from build123d import *

# Parameters (mm, degrees)
BOSS_EXTRUDE2_DEPTH   = 6.35
BOSS_EXTRUDE2_2_DEPTH = 6.35
BOSS_EXTRUDE3_DEPTH   = 12.7
CUT_EXTRUDE2_REACH    = 189.943
SKETCH3_R             = 1.397
CUT_EXTRUDE3_REACH    = 184.986
SKETCH4_R             = 1.35255
SKETCH5_R             = 1.75
CUT_EXTRUDE5_DEPTH    = 24


with BuildPart() as part:
    # Sketch1 → Boss-Extrude2 (new body)
    with BuildSketch(Plane(origin=(0, 0, 0), x_dir=(1, 0, 0), z_dir=(0, 1, 0))):
        Polygon((12.7, 68.58), (40.64, 68.58), (40.64, 78.74), (0, 78.74), (0, 12.7), (12.7, 12.7), align=None)
    extrude(amount=BOSS_EXTRUDE2_DEPTH)



with BuildPart() as body_2:
    # Sketch1 → Boss-Extrude2 2 (new body)
    with BuildSketch(Plane(origin=(0, 0, 0), x_dir=(1, 0, 0), z_dir=(0, 1, 0))):
        Polygon((157.48, 68.58), (157.48, 12.7), (170.18, 12.7), (170.18, 78.74), (129.54, 78.74), (129.54, 68.58), align=None)
    extrude(amount=BOSS_EXTRUDE2_2_DEPTH)


with BuildPart() as part_1:
    add(part.part)

    add(body_2.part)  # Boss-Extrude3 merges body 2
    # Sketch1_3 → Boss-Extrude3 (add)
    with BuildSketch(Plane(origin=(0, 0, 0), x_dir=(1, 0, 0), z_dir=(0, 1, 0))):
        Polygon((157.48, 12.7), (12.7, 12.7), (0, 12.7), (0, 0), (170.18, 0), (170.18, 12.7), align=None)
    extrude(amount=BOSS_EXTRUDE3_DEPTH)

    # Sketch3 → Cut-Extrude2 (cut, up to next)
    with BuildSketch(Plane(origin=(0, 12.7, 0), x_dir=(1, 0, 0), z_dir=(0, 1, 0)), mode=Mode.PRIVATE) as cut_extrude2_sk1:
        with Locations(Location((75.565, 4.7625, 0), (0, 0, 270))):
            Circle(SKETCH3_R)
    cut_extrude2_tool1 = extrude(cut_extrude2_sk1.sketch, amount=-CUT_EXTRUDE2_REACH, mode=Mode.PRIVATE) & part_1.part
    # Sketch3 → Cut-Extrude2 (cut, up to next)
    with BuildSketch(Plane(origin=(0, 12.7, 0), x_dir=(1, 0, 0), z_dir=(0, 1, 0)), mode=Mode.PRIVATE) as cut_extrude2_sk2:
        with Locations(Location((94.615, 7.9375, 0), (0, 0, 270))):
            Circle(SKETCH3_R)
    cut_extrude2_tool2 = extrude(cut_extrude2_sk2.sketch, amount=-CUT_EXTRUDE2_REACH, mode=Mode.PRIVATE) & part_1.part
    add(cut_extrude2_tool1.solids().sort_by_distance((75.565, 12.7, -4.7625))[0], mode=Mode.SUBTRACT)
    add(cut_extrude2_tool2.solids().sort_by_distance((94.615, 12.7, -7.9375))[0], mode=Mode.SUBTRACT)

    # Sketch4 → Cut-Extrude3 (cut, up to next)
    with BuildSketch(Plane(origin=(0, 0, -12.7), x_dir=(-1, 0, 0), z_dir=(0, 0, -1)), mode=Mode.PRIVATE) as cut_extrude3_sk1:
        with Locations((-87.4776, 3.175)):
            Circle(SKETCH4_R)
    cut_extrude3_tool1 = extrude(cut_extrude3_sk1.sketch, amount=-CUT_EXTRUDE3_REACH, mode=Mode.PRIVATE) & part_1.part
    # Sketch4 → Cut-Extrude3 (cut, up to next)
    with BuildSketch(Plane(origin=(0, 0, -12.7), x_dir=(-1, 0, 0), z_dir=(0, 0, -1)), mode=Mode.PRIVATE) as cut_extrude3_sk2:
        with Locations((-79.546452542, 9.525)):
            Circle(SKETCH4_R)
    cut_extrude3_tool2 = extrude(cut_extrude3_sk2.sketch, amount=-CUT_EXTRUDE3_REACH, mode=Mode.PRIVATE) & part_1.part
    add(cut_extrude3_tool1.solids().sort_by_distance((87.4776, 3.175, -12.7))[0], mode=Mode.SUBTRACT)
    add(cut_extrude3_tool2.solids().sort_by_distance((79.546453, 9.525, -12.7))[0], mode=Mode.SUBTRACT)

    # Sketch5 → Cut-Extrude5 (cut)
    with BuildSketch(Plane(origin=(0, 0, -12.7), x_dir=(-1, 0, 0), z_dir=(0, 0, -1))):
        with Locations((-88.265, 9.525)):
            Circle(SKETCH5_R)
        with Locations((-81.915, 3.175)):
            Circle(SKETCH5_R)
    extrude(amount=-CUT_EXTRUDE5_DEPTH, mode=Mode.SUBTRACT)


solid = part_1.part
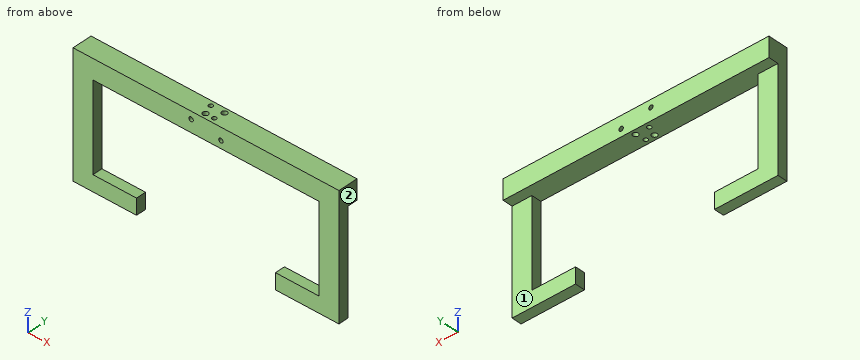
Build history of the part. All positions in model axes, mm. Face numbers are marked on the shaded views. A direction names the side the tool comes from. Give positions to 0.01 mm unless a question says otherwise; leave off trailing zeros. Order: outer loops, then holes, each group sorted by start corner. A loop starts at its lowest first (then second) coordinate and runs counter-clockwise, first axis right, second up. Notation, with made-up numbers: M 38,63 L 82,63 A12 ccw 82,68 Z; hole C -37,11 d2. An arc over 180 degrees is marked long. Use one line per item in the form item = value.
Q1. Slice it at B-B, the plane z = -74. Write the cut outline in (x, y), and give its area (3 significant figures).
Conclusion:
outline = M 0,0 L 40.64,0 L 40.64,6.35 L 0,6.35 Z; M 129.54,0 L 170.18,0 L 170.18,6.35 L 129.54,6.35 Z
area = 516 mm2
Q2. Slice it at C-C, the plane x = 104.5. Write the cut outline in (y, z), and give its area (3 significant figures).
Conclusion:
outline = M 0,-12.7 L 12.7,-12.7 L 12.7,0 L 0,0 Z
area = 161 mm2
Q3. Wall check: probe 1 along Z at (x, y) = (17, 3.25); probe 2 along X at (y, z) = (1.75, -42); probe 3 along X at (y, z) = (9, -5). Give the ranges that are in metal, low to high.
Conclusion:
probe_1 = -78.74 to -68.58, -12.7 to 0
probe_2 = 0 to 12.7, 157.48 to 170.18
probe_3 = 0 to 74.19, 76.94 to 78.3, 80.79 to 86.6, 89.93 to 170.18
Q4. Slice it at A-A, the plane x = 153. Write the cut outline in (y, z), and give its area (3 significant figures).
Conclusion:
outline = M 0,-78.74 L 6.35,-78.74 L 6.35,-68.58 L 0,-68.58 Z; M 0,-12.7 L 12.7,-12.7 L 12.7,0 L 0,0 Z
area = 226 mm2
Q5. Which spindle directions (+Z, -Z, +X, -X, +Y, -Y) get a long thin tool onto all of the face, cutting with end or side? Do the marked faces 1 and 2. Say none if no direction does.
Conclusion:
face_1 = -Z, +X, -X, +Y
face_2 = +Z, -Z, +X, +Y, -Y
Q6. Pin check, flat tips, straight feed: P1, Ø3, axis at x = 130, z = -15.5, coming from the +Y side; P2, Ø4.5, axis at x = 81.915, y = 3.175, coming from the -Z side. Stop position of each tip, or through.
Conclusion:
P1 = through
P2 = -12.7
